```python
from build123d import *

# Parameters (mm, degrees)
F0_W     = 152.4
F0_H     = 304.8
F1_DEPTH = 6.35
F2_W     = 6.35
F2_H     = 12.7
F2_W_2   = 48.26
F2_H_2   = 60.96
F2_W_3   = 25.4
F2_H_3   = 7.9375
F3_DEPTH = 6.351
F4_W     = 6.35
F4_H     = 12.7
F5_DEPTH = 25.4


with BuildPart() as f1:
    # F0 (on Top) → F1 (new body)
    with BuildSketch(Plane.XY):
        with Locations((76.2, 152.4)):
            Rectangle(F0_W, F0_H)
    extrude(amount=F1_DEPTH)

    # F2 (on face) → F3 (cut, through all)
    with BuildSketch(Plane.XY.offset(6.35)):
        with Locations((123.825, 50.8)):
            Rectangle(F2_W, F2_H)
        with Locations((47.625, 50.8)):
            Rectangle(F2_W, F2_H)
        with Locations((123.825, 101.6)):
            Rectangle(F2_W, F2_H)
        with Locations((47.625, 101.6)):
            Rectangle(F2_W, F2_H)
        with Locations((123.825, 190.5)):
            Rectangle(F2_W, F2_H)
        with Locations((85.725, 190.5)):
            Rectangle(F2_W, F2_H)
        with Locations((109.22, 253.6825)):
            Rectangle(F2_W_2, F2_H_2)
        with Locations((44.45, 190.50635)):
            Rectangle(F2_W_3, F2_H_3)
        Polygon((25.4, 159.5628), (25.4, 133.8072), (70.612, 133.8072), (70.612, 159.5628), (74.93, 159.5628), (74.93, 170.9928), (21.082, 170.9928), (21.082, 159.5628), align=None)
        with Locations((41.91, 253.6825)):
            Rectangle(F2_W_2, F2_H_2)
    extrude(amount=-F3_DEPTH, mode=Mode.SUBTRACT)

    # F4 (on face) → F5 (cut)
    with BuildSketch(Plane.XY.offset(6.35)):
        with Locations((139.920227, 50.8)):
            Rectangle(F4_W, F4_H)
        with Locations((139.920227, 101.6)):
            Rectangle(F4_W, F4_H)
    extrude(amount=-F5_DEPTH, mode=Mode.SUBTRACT)


solid = f1.part
```
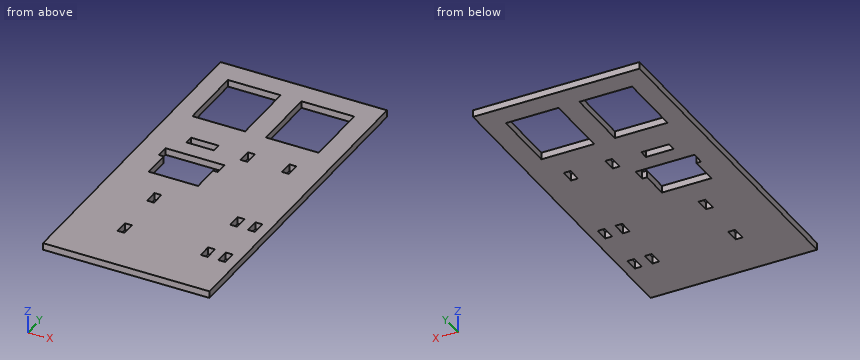
Work out the finished part from the listing and answer in its coordinate system (mm). Coordinates: 2 decimals unless noted, no trailing zeros. Loops run counter-clockwise (first coordinate to the right, second up) from the corner with the lowest first, then second, coordinate; pieces in that order, holes last. Notation, with made-up numbers: (45, -1.5) -> (73, -1.5) arc R20 cw to (73, 25.5) -> close; hole circle Ø2 at (57, 42.25). An arc over 180 degrees is marked (long way). Answer as CSV lines item,"result".
Q1. The part is cut by section D-D on x = 62. Write down the section's boundary in (y, z).
Findings:
outline,"(0, 0) -> (133.81, 0) -> (133.81, 6.35) -> (0, 6.35) -> close; (170.99, 0) -> (223.2, 0) -> (223.2, 6.35) -> (170.99, 6.35) -> close; (284.16, 0) -> (304.8, 0) -> (304.8, 6.35) -> (284.16, 6.35) -> close"
Q2. Find the intervals of material crossed by probe 1 along X at (y, z) = (257, 4); probe 2 along Y at (x, z) = (36.5, 6); probe 3 along X at (y, z) = (97, 5.75), in increasing order.
Findings:
probe 1,"x = 0 to 17.78, 66.04 to 85.09, 133.35 to 152.4"
probe 2,"y = 0 to 133.81, 170.99 to 186.54, 194.48 to 223.2, 284.16 to 304.8"
probe 3,"x = 0 to 44.45, 50.8 to 120.65, 127 to 136.75, 143.1 to 152.4"
Q3. The part is cut by section A-A on x = 98.5. Write down the section's boundary in (y, z).
Findings:
outline,"(0, 0) -> (223.2, 0) -> (223.2, 6.35) -> (0, 6.35) -> close; (284.16, 0) -> (304.8, 0) -> (304.8, 6.35) -> (284.16, 6.35) -> close"
Q4. The part is cut by section C-C on y = 141. Write down the section's boundary in (x, z).
Findings:
outline,"(0, 0) -> (25.4, 0) -> (25.4, 6.35) -> (0, 6.35) -> close; (70.61, 0) -> (152.4, 0) -> (152.4, 6.35) -> (70.61, 6.35) -> close"
Q5. The part is cut by section B-B on y = 227. Write down the section's boundary in (x, z).
Findings:
outline,"(0, 0) -> (17.78, 0) -> (17.78, 6.35) -> (0, 6.35) -> close; (66.04, 0) -> (85.09, 0) -> (85.09, 6.35) -> (66.04, 6.35) -> close; (133.35, 0) -> (152.4, 0) -> (152.4, 6.35) -> (133.35, 6.35) -> close"
